from build123d import *

# Parameters (mm, degrees)
F0_W     = 19.05
F0_H     = 1.8288
F0_R     = 0.3175
F1_DEPTH = 0.762
F0_H_2   = 2.2606
F2_DEPTH = 2.286


with BuildPart() as f1:
    # F0 (on Top) → F1 (new body)
    with BuildSketch(Plane.XY):
        Rectangle(F0_W, F0_H)
        with Locations((-6.35, 0)):
            Circle(F0_R, mode=Mode.SUBTRACT)
        with Locations((6.35, 0)):
            Circle(F0_R, mode=Mode.SUBTRACT)
    extrude(amount=F1_DEPTH)

    # F0 (on Top) → F2 (join)
    with BuildSketch(Plane.XY):
        with Locations((0, -2.0447)):
            Rectangle(F0_W, F0_H_2)
        with Locations((0, 2.0447)):
            Rectangle(F0_W, F0_H_2)
    extrude(amount=F2_DEPTH)


solid = f1.part
The model under review builds one solid part; all positions refer to its coordinate system, in mm. A direction names the side the tool comes from. Coordinates: 2 decimals unless noted, no trailing zeros. Loops run counter-clockwise (first coordinate to the right, second up) from the corner with the lowest first, then second, coordinate; pieces in that order, holes last.
(1) Consider section C-C, the plane x = 6.35. Give the boundary of the cut face in (y, z) (1 decimal), plus the area to 3 significant figures.
Determined:
outline: (-3.2, 0) - (-0.3, 0) - (-0.3, 0.8) - (-0.9, 0.8) - (-0.9, 2.3) - (-3.2, 2.3) - close; (0.3, 0) - (3.2, 0) - (3.2, 2.3) - (0.9, 2.3) - (0.9, 0.8) - (0.3, 0.8) - close
area: 11.2 mm2
(2) Consider section B-B, the plane z = 1.9. Give the boundary of the cut face in (x, y) (3 decimals), plus the area to 3 significant figures.
Determined:
outline: (-9.525, -3.175) - (9.525, -3.175) - (9.525, -0.914) - (-9.525, -0.914) - close; (-9.525, 0.914) - (9.525, 0.914) - (9.525, 3.175) - (-9.525, 3.175) - close
area: 86.1 mm2
(3) Tool access review of faces 1 (the flat face through (0, 2, 2.286)), 2 (the flat face through (0, -0.914, 2)): name each direction out of +Z, -Z, +X, -X, +Y, -Y from which nothing blocks a thin tool from reaching the whole face with its end or side.
Determined:
face 1: +Z, +X, -X, +Y, -Y
face 2: +Z, +X, -X
(4) Consider section A-A, the plane y = 0. Give the boundary of the cut face in (x, z) (1 decimal), plus the area to 3 significant figures.
Determined:
outline: (-9.5, 0) - (-6.7, 0) - (-6.7, 0.8) - (-9.5, 0.8) - close; (-6, 0) - (6, 0) - (6, 0.8) - (-6, 0.8) - close; (6.7, 0) - (9.5, 0) - (9.5, 0.8) - (6.7, 0.8) - close
area: 13.5 mm2
(5) Insertion check: P1, Ø1, axis at x = 7.5, y = 2, coming from the -Z side. The pin has a flat end and moves straight along its axis. Give the tip position at first contact, or say it passes through.
Determined:
P1: stops at z = 0
(6) Consider section D-D, the plane x = 1. Give the boundary of the cut face in (y, z) (3 decimals), plus the area to 3 significant figures.
Determined:
outline: (-3.175, 0) - (3.175, 0) - (3.175, 2.286) - (0.914, 2.286) - (0.914, 0.762) - (-0.914, 0.762) - (-0.914, 2.286) - (-3.175, 2.286) - close
area: 11.7 mm2
(7) Draft analysis for pull direction Y (two halves, no side actions). For faces 3 (the flat face through (0, -3.175, 1)), 4 (the flat face through (0, 0, 0.762)), 5 (the flat face through (0, 0, 0)), state which applies: +Y half, -Y half, draft (parallel to the pull), parting line (faces both ways), or undercut.
Determined:
face 3: -Y half
face 4: undercut
face 5: draft
(8) Wall thickness on L1, parallel to Y at x = 2, z = 1.2 (3 decimals); L2, parallel to Y at x = -6.35, z = 0.65 (1 decimal): over which ranges is each line inside the solid? List them lowest first.
Determined:
L1: y = -3.175 to -0.914, 0.914 to 3.175
L2: y = -3.2 to -0.3, 0.3 to 3.2
